```python
from build123d import *

# Parameters (mm, degrees)
F0_R     = 2
F1_DEPTH = 20
F2_R     = 2


with BuildPart() as f1:
    # F0 (on Right) → F1 (new body)
    with BuildSketch(Plane.YZ):
        with BuildLine():
            ThreePointArc((7, 24.021733), (0, 45.768528), (-7, 24.021733))
            Line((-7, 24.021733), (-7, -21.484678))
            ThreePointArc((-7, -21.484678), (0, -43.231472), (7, -21.484678))
            Line((7, -21.484678), (7, 24.021733))
        make_face()
        with Locations((0, -31.231472)):
            Circle(F0_R, mode=Mode.SUBTRACT)
        with Locations((0, 33.768528)):
            Circle(F0_R, mode=Mode.SUBTRACT)
    extrude(amount=F1_DEPTH)

    # F2
    f2_edges = [f1.edges().sort_by_distance(p)[0] for p in [
        (0, -7, 1.268528),
        (0, 0, -43.231472),
        (0, 7, 1.268528),
        (0, 0, 45.768528),
    ]]
    fillet(f2_edges, radius=F2_R)


solid = f1.part
```
The listing builds one solid part. Answer for the finished solid, in the listing's coordinates (mm). A direction names the side the tool comes from. Give positions to 0.01 mm unless a question says otherwise; leave off trailing zeros. Order: outer loops, then holes, each group sorted by start corner. A loop starts at its lowest first (then second) coordinate and runs counter-clockwise, first axis right, second up. Notation, with made-up numbers: M 11,62 L 60,62 A26 ccw 60,97 Z; hole C 40.25,12 d2. An arc over 180 degrees is marked long. Put each result on its own line as item: value. Start each with the question number.
Item 1: The part is cut by section B-B, the plane x = 3.5. Determine the outline of the cut face in (y, z), and give its area (3 significant figures).
Item 2: Which of the six approach directions +Z, -Z, +X, -X, +Y, -Y give full straight-line access (tool end or side, diameter ignored) to faces 1 (the face through (0.6, 6.43, 1.6)), 2 (the face through (11, 7, 1)), 3 (the face through (10.874, -0.423, -43.224)), 4 (the face through (0.6, -6.43, 0.93))?
Item 3: Find the intervals of material crossed by line 1 along Z through (x, y) = (9.75, 0); line 2 along Y through (x, z) = (9, 18.5); line 3 along X through (y, z) = (-5.25, -22), in increasing order.
Item 4: The part is cut by section A-A, the plane y = 0. Determine the outline of the cut face in (x, z).
Item 5: For a pull along Y with two mould halves and no side action, classify faces 5 (the face through (0, 0, 2)), 6 (the face through (10.87, 0.42, 45.76)), 7 (the face through (11, -7, 2)), 8 (the face through (9.86, -0.434, -33.184)) as +Y half, -Y half, draft (parallel to the pull), parting line (faces both ways), or undercut.
Item 6: Flat-ended cylindrical pins translate along their axes: P1, Ø8, axis at x = 14.5, z = -3, coming from the +Y side; P2, Ø8, axis at x = 6, y = 8, coming from the +Z side; P3, Ø4, axis at x = 4.5, z = 24.5, coming from the -Y side. Find the tip coordinate at first contact, or state that the pin passes through.
Item 7: The part is cut by section C-C, the plane z = 7.5. Determine the outline of the cut face in (x, y), and give its area (3 significant figures).
Answer key:
1. outline: M -7,-21.48 A12 ccw long 7,-21.48 L 7,24.02 A12 ccw long -7,24.02 Z; hole C 0,-31.23 d4; hole C 0,33.77 d4
1. area: 1,470 mm²
2. face 1: -X, +Y
2. face 2: +X, -X, +Y
2. face 3: +X, -X
2. face 4: -X, -Y
3. line 1: z = -43.23 to -33.23, -29.23 to 31.77, 35.77 to 45.77
3. line 2: y = -7 to 7
3. line 3: x = 0.02 to 20
4. outline: M 0,-41.23 A2 ccw 2,-43.23 L 20,-43.23 L 20,-33.23 L 0,-33.23 Z; M 0,-29.23 L 20,-29.23 L 20,31.77 L 0,31.77 Z; M 0,35.77 L 20,35.77 L 20,45.77 L 2,45.77 A2 ccw 0,43.77 Z
5. face 5: draft
5. face 6: parting line
5. face 7: -Y half
5. face 8: undercut
6. P1: stops at y = 7
6. P2: stops at z = 45.08
6. P3: stops at y = -9.55
7. outline: M 0,-5 A2 ccw 2,-7 L 20,-7 L 20,7 L 2,7 A2 ccw 0,5 Z
7. area: 278 mm²
